```python
from build123d import *

# Parameters (mm, degrees)
SKIZZE1_R                                  = 38.5
AUFSATZ_LINEAR_AUSTRAGEN1_DEPTH            = 39
SCHNITT_LINEAR_AUSTRAGEN1_DEPTH            = 32.5
SKIZZE3_R                                  = 26.075
SCHNITT_LINEAR_AUSTRAGEN2_DEPTH            = 67.973875504
F_2_5_2_5_DURCHMESSER_BOHRUNG1_D           = 2.5
F_2_5_2_5_DURCHMESSER_BOHRUNG1_CSINK_D     = 3.5
F_2_5_2_5_DURCHMESSER_BOHRUNG1_CSINK_ANGLE = 90
F_2_5_2_5_DURCHMESSER_BOHRUNG2_D           = 2.5
F_2_5_2_5_DURCHMESSER_BOHRUNG2_DEPTH       = 15
F_2_5_2_5_DURCHMESSER_BOHRUNG2_CSINK_D     = 3.5
F_2_5_2_5_DURCHMESSER_BOHRUNG2_CSINK_ANGLE = 90
F_2_5_2_5_DURCHMESSER_BOHRUNG2_TIP         = 0.751075774
FASE1_SIZE                                 = 0.5


with BuildPart() as part:
    # Skizze1 → Aufsatz-Linear austragen1 (new body)
    with BuildSketch(Plane(origin=(0, 0, 0), x_dir=(1, 0, 0), z_dir=(0, 1, 0))):
        with Locations(Location((0, 0, 0), (0, 0, 270))):
            Circle(SKIZZE1_R)
    extrude(amount=AUFSATZ_LINEAR_AUSTRAGEN1_DEPTH)

    # Skizze2 → Schnitt-Linear austragen1 (cut)
    with BuildSketch(Plane(origin=(0, 39, 0), x_dir=(1, 0, 0), z_dir=(0, 1, 0))):
        with BuildLine():
            ThreePointArc((4.489203024, 32.188461538), (0, 37), (-4.489203024, 32.188461538))
            ThreePointArc((-4.489203024, 32.188461538), (-6.340435466, 31.875521613), (-8.170508153, 31.45620442))
            ThreePointArc((-8.170508153, 31.45620442), (-14.159286998, 34.183542703), (-16.465473735, 28.020317177))
            ThreePointArc((-16.465473735, 28.020317177), (-18.056032573, 27.0227624), (-19.58633353, 25.93502533))
            ThreePointArc((-19.58633353, 25.93502533), (-26.162950904, 26.162950904), (-25.93502533, 19.58633353))
            ThreePointArc((-25.93502533, 19.58633353), (-27.0227624, 18.056032573), (-28.020317177, 16.465473735))
            ThreePointArc((-28.020317177, 16.465473735), (-34.183542703, 14.159286998), (-31.45620442, 8.170508153))
            ThreePointArc((-31.45620442, 8.170508153), (-31.875521613, 6.340435466), (-32.188461538, 4.489203024))
            ThreePointArc((-32.188461538, 4.489203024), (-37, 0), (-32.188461538, -4.489203024))
            ThreePointArc((-32.188461538, -4.489203024), (-31.875521613, -6.340435466), (-31.45620442, -8.170508153))
            ThreePointArc((-31.45620442, -8.170508153), (-34.183542703, -14.159286998), (-28.020317177, -16.465473735))
            ThreePointArc((-28.020317177, -16.465473735), (-27.0227624, -18.056032573), (-25.93502533, -19.58633353))
            ThreePointArc((-25.93502533, -19.58633353), (-26.162950904, -26.162950904), (-19.58633353, -25.93502533))
            ThreePointArc((-19.58633353, -25.93502533), (-18.056032573, -27.0227624), (-16.465473735, -28.020317177))
            ThreePointArc((-16.465473735, -28.020317177), (-14.159286998, -34.183542703), (-8.170508153, -31.45620442))
            ThreePointArc((-8.170508153, -31.45620442), (-6.340435466, -31.875521613), (-4.489203024, -32.188461538))
            ThreePointArc((-4.489203024, -32.188461538), (0, -37), (4.489203024, -32.188461538))
            ThreePointArc((4.489203024, -32.188461538), (6.340435466, -31.875521613), (8.170508153, -31.45620442))
            ThreePointArc((8.170508153, -31.45620442), (14.159286998, -34.183542703), (16.465473735, -28.020317177))
            ThreePointArc((16.465473735, -28.020317177), (18.056032573, -27.0227624), (19.58633353, -25.93502533))
            ThreePointArc((19.58633353, -25.93502533), (26.162950904, -26.162950904), (25.93502533, -19.58633353))
            ThreePointArc((25.93502533, -19.58633353), (27.0227624, -18.056032573), (28.020317177, -16.465473735))
            ThreePointArc((28.020317177, -16.465473735), (34.183542703, -14.159286998), (31.45620442, -8.170508153))
            ThreePointArc((31.45620442, -8.170508153), (31.875521613, -6.340435466), (32.188461538, -4.489203024))
            ThreePointArc((32.188461538, -4.489203024), (37, 0), (32.188461538, 4.489203024))
            ThreePointArc((32.188461538, 4.489203024), (31.875521613, 6.340435466), (31.45620442, 8.170508153))
            ThreePointArc((31.45620442, 8.170508153), (34.183542703, 14.159286998), (28.020317177, 16.465473735))
            ThreePointArc((28.020317177, 16.465473735), (27.0227624, 18.056032573), (25.93502533, 19.58633353))
            ThreePointArc((25.93502533, 19.58633353), (26.162950904, 26.162950904), (19.58633353, 25.93502533))
            ThreePointArc((19.58633353, 25.93502533), (18.056032573, 27.0227624), (16.465473735, 28.020317177))
            ThreePointArc((16.465473735, 28.020317177), (14.159286998, 34.183542703), (8.170508153, 31.45620442))
            ThreePointArc((8.170508153, 31.45620442), (6.340435466, 31.875521613), (4.489203024, 32.188461538))
        make_face()
    extrude(amount=-SCHNITT_LINEAR_AUSTRAGEN1_DEPTH, mode=Mode.SUBTRACT)

    # Skizze3 → Schnitt-Linear austragen2 (cut, through all)
    with BuildSketch(Plane.XZ):
        with Locations(Location((0, 0, 0), (0, 0, 270))):
            Circle(SKIZZE3_R)
    extrude(amount=-SCHNITT_LINEAR_AUSTRAGEN2_DEPTH, mode=Mode.SUBTRACT)

    # Ø2.5 (2.5) Durchmesser Bohrung1 (through all)
    with Locations(Plane(origin=(0, 6.5, 0), x_dir=(1, 0, 0), z_dir=(0, 1, 0))):
        with Locations((0, 32.5), (12.437211552, 30.026084807), (22.980970389, 22.980970389), (30.026084807, 12.437211552), (32.5, 0), (30.026084807, -12.437211552), (22.980970389, -22.980970389), (12.437211552, -30.026084807), (0, -32.5), (-12.437211552, -30.026084807), (-22.980970389, -22.980970389), (-30.026084807, -12.437211552), (-32.5, 0), (-30.026084807, 12.437211552), (-22.980970389, 22.980970389), (-12.437211552, 30.026084807)):
            CounterSinkHole(F_2_5_2_5_DURCHMESSER_BOHRUNG1_D / 2, F_2_5_2_5_DURCHMESSER_BOHRUNG1_CSINK_D / 2, counter_sink_angle=F_2_5_2_5_DURCHMESSER_BOHRUNG1_CSINK_ANGLE)

    # Ø2.5 (2.5) Durchmesser Bohrung2
    with Locations(Plane(origin=(0, 39, 0), x_dir=(1, 0, 0), z_dir=(0, 1, 0))):
        with Locations((-34.827105043, -6.879153607), (-6.879153607, 34.827105043), (34.827105043, 6.879153607), (6.879153607, -34.827105043)):
            CounterSinkHole(F_2_5_2_5_DURCHMESSER_BOHRUNG2_D / 2, F_2_5_2_5_DURCHMESSER_BOHRUNG2_CSINK_D / 2, depth=F_2_5_2_5_DURCHMESSER_BOHRUNG2_DEPTH, counter_sink_angle=F_2_5_2_5_DURCHMESSER_BOHRUNG2_CSINK_ANGLE)
            with Locations((0, 0, -(F_2_5_2_5_DURCHMESSER_BOHRUNG2_DEPTH + F_2_5_2_5_DURCHMESSER_BOHRUNG2_TIP / 2))):  # 118° drill point
                Cone(0, F_2_5_2_5_DURCHMESSER_BOHRUNG2_D / 2, F_2_5_2_5_DURCHMESSER_BOHRUNG2_TIP, mode=Mode.SUBTRACT)

    # Fase1
    fase1_edges = [part.edges().sort_by_distance(p)[0] for p in [
        (0, 0, 26.075),
    ]]
    chamfer(fase1_edges, length=FASE1_SIZE)


solid = part.part
```
Could you check a few things on this model? Use its own coordinates, in mm. A direction names the side the tool comes from. Give positions to 0.01 mm unless a question says otherwise; leave off trailing zeros. Order: outer loops, then holes, each group sorted by start corner. A loop starts at its lowest first (then second) coordinate and runs counter-clockwise, first axis right, second up.
Q1. If I drill on line 1 along X through (y, z) = (28, 12); line 2 along Z through (x, y) = (0.5, 3); line 3 along Z through (x, y) = (-33.5, 12.5), over which ranges is the centre line in solid material (lowest first)?
Q2. Suppose I cut it at A-A, the plane z = 0. Write out the boundary of the cut face in (x, y) (3 decimals), and give its area (3 significant figures).
Q3. Suppose I cut it at C-C, the plane y = 30. Count the separate pieces of the cut face and the enclosed holes in it, and give its area (3 significant figures).
Q4. For faces 1 (the cylindrical face through (18.078, 22.978, -27.008)), 2 (the cylindrical face through (23.25, 2.96, 24.2)), which set-ups out of +Z, -Z, +X, -X, +Y, -Y let a thin tool reach every point of the face, with its end or its side?
Q5. I'm going to push flat-ended pins straight in: P1, Ø8, axis at x = 11, y = 29, coming from the +Z side; P2, Ø3, axis at x = -34.83, z = 6.88, coming from the +Y side; P3, Ø8, axis at y = 30, z = -7, coming from the +X side. Where does each tip first touch, or does it pass through?
Solution:
1. line 1: x = -36.58 to -34.5, 34.5 to 36.58
1. line 2: z = -38.5 to -33.65, -31.35 to -26.07, 26.07 to 31.35, 33.65 to 38.5
1. line 3: z = -18.97 to -15.3, -9.58 to -4.39, 4.39 to 9.58, 15.3 to 18.97
2. outline: (-38.5, 0) - (-33.75, 0) - (-33.75, 6) - (-34.25, 6.5) - (-37, 6.5) - (-37, 39) - (-38.5, 39) - close; (-31.25, 0) - (-26.575, 0) - (-26.075, 0.5) - (-26.075, 6.5) - (-30.75, 6.5) - (-31.25, 6) - close; (26.075, 0.5) - (26.575, 0) - (31.25, 0) - (31.25, 6) - (30.75, 6.5) - (26.075, 6.5) - close; (33.75, 0) - (38.5, 0) - (38.5, 39) - (37, 39) - (37, 6.5) - (34.25, 6.5) - (33.75, 6) - close
2. area: 226 mm2
3. separate pieces: 1
3. enclosed holes: 5
3. area: 795 mm2
4. face 1: +Y
4. face 2: +Y, -Y
5. P1: stops at z = 37.86
5. P2: stops at y = 38.75
5. P3: stops at x = 38.38
